Could you check a few things on this model? Use its own coordinates, in mm. Face numbers are marked on the shaded views. A direction names the side the tool comes from. Coordinates: 2 decimals unless noted, no trailing zeros. Write each loop counter-clockwise with the first axis right and the second up, starting at its lowest first coordinate (ties: lowest second). Pieces come first, ordered by that corner, then holes. Notation, with made-up numbers: M -2.5,7 L 38.5,7 A25 ccw 38.5,21 Z; hole C 57,40 d11. An arc over 180 degrees is marked long. Write item = value, one per line.
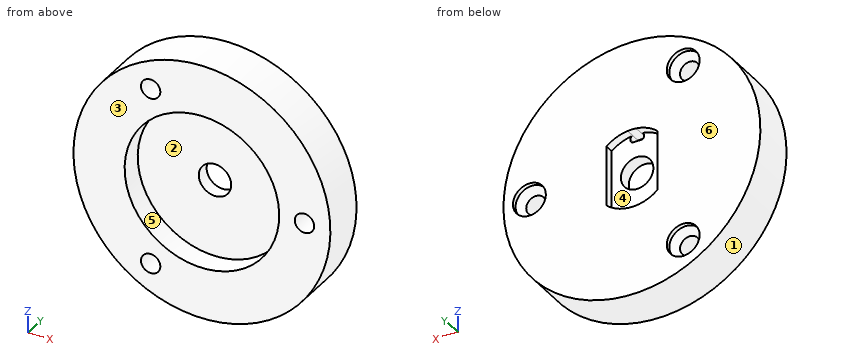
```python
from build123d import *

# Parameters (mm, degrees)
SKETCH_714_R           = 3.6
CUT_EXTRUDE_1503_DEPTH = 2
CUT_EXTRUDE_1558_DEPTH = 4
SKETCH_1765_R          = 2.15
CUT_EXTRUDE_2399_DEPTH = 42.527099586
SKETCH_3_5_R           = 3.65
CUT_EXTRUDE_2433_DEPTH = 0.5
CHAMFER_3010_SIZE      = 2


with BuildPart() as part:
    # Sketch 314 → Повернуть1 (revolve)
    with BuildSketch(Plane.XY, mode=Mode.PRIVATE) as revolve_1_sk:
        Polygon((3.6, 10), (28.5, 10), (28.5, 0), (17.15, 0), (17.15, 5), (3.6, 5), align=None)
    revolve(revolve_1_sk.sketch.rotate(Axis((0, 24.786794377, 0), (0, -1, 0)), 90), axis=Axis((0, 24.786794377, 0), (0, -1, 0)))

    # Sketch 714 → Cut-Extrude 1503 (cut)
    # profile 1 of 2: a face of its own
    with BuildSketch(Plane(origin=(0, 10, 0), x_dir=(1, 0, 0), z_dir=(0, 1, 0))):
        with BuildLine():
            ThreePointArc((-1.5, -7.78), (-1.330121933, -7.369878067), (-0.92, -7.2))
            Line((-0.92, -7.2), (0.92, -7.2))
            ThreePointArc((0.92, -7.2), (1.330121933, -7.369878067), (1.5, -7.78))
            Line((1.5, -7.78), (1.5, -8.082233602))
            ThreePointArc((1.5, -8.082233602), (1.341523495, -8.496233679), (0.947109471, -8.6985909))
            ThreePointArc((0.947109471, -8.6985909), (3.449320455, -8.041435717), (5.65, -6.681317235))
            Line((5.65, -6.681317235), (5.65, 6.681317235))
            ThreePointArc((5.65, 6.681317235), (0, 8.75), (-5.65, 6.681317235))
            Line((-5.65, 6.681317235), (-5.65, -6.681317235))
            ThreePointArc((-5.65, -6.681317235), (-3.449320455, -8.041435717), (-0.947109471, -8.6985909))
            ThreePointArc((-0.947109471, -8.6985909), (-1.341523495, -8.496233679), (-1.5, -8.082233602))
            Line((-1.5, -8.082233602), (-1.5, -7.78))
        make_face()
        with Locations(Location((0, 0, 0), (0, 0, 270))):
            Circle(SKETCH_714_R, mode=Mode.SUBTRACT)
    # profile 2 of 2: a face of its own
    with BuildSketch(Plane(origin=(0, 10, 0), x_dir=(1, 0, 0), z_dir=(0, 1, 0))):
        with BuildLine():
            ThreePointArc((-1.5, -7.78), (-1.330121933, -7.369878067), (-0.92, -7.2))
            Line((-0.92, -7.2), (0.92, -7.2))
            ThreePointArc((0.92, -7.2), (1.330121933, -7.369878067), (1.5, -7.78))
            Line((1.5, -7.78), (1.5, -8.082233602))
            ThreePointArc((1.5, -8.082233602), (1.341523495, -8.496233679), (0.947109471, -8.6985909))
            ThreePointArc((0.947109471, -8.6985909), (0, -8.75), (-0.947109471, -8.6985909))
            ThreePointArc((-0.947109471, -8.6985909), (-1.341523495, -8.496233679), (-1.5, -8.082233602))
            Line((-1.5, -8.082233602), (-1.5, -7.78))
        make_face()
    extrude(amount=-CUT_EXTRUDE_1503_DEPTH, mode=Mode.SUBTRACT)

    # Эскиз2<3> → Cut-Extrude 1558 (cut)
    with BuildSketch(Plane(origin=(0, 10, 0), x_dir=(1, 0, 0), z_dir=(0, 1, 0))):
        with BuildLine():
            ThreePointArc((-1.5, -7.78), (-1.330121933, -7.369878067), (-0.92, -7.2))
            Line((-0.92, -7.2), (0.92, -7.2))
            ThreePointArc((0.92, -7.2), (1.330121933, -7.369878067), (1.5, -7.78))
            Line((1.5, -7.78), (1.5, -8.082233602))
            ThreePointArc((1.5, -8.082233602), (1.341523495, -8.496233679), (0.947109471, -8.6985909))
            ThreePointArc((0.947109471, -8.6985909), (0, -8.75), (-0.947109471, -8.6985909))
            ThreePointArc((-0.947109471, -8.6985909), (-1.341523495, -8.496233679), (-1.5, -8.082233602))
            Line((-1.5, -8.082233602), (-1.5, -7.78))
        make_face()
    extrude(amount=-CUT_EXTRUDE_1558_DEPTH, mode=Mode.SUBTRACT)

    # Sketch 1765 → Cut-Extrude 2399 (cut, through all)
    with BuildSketch(Plane(origin=(0, 10, 0), x_dir=(1, 0, 0), z_dir=(0, 1, 0))):
        with Locations(Location((22.75, 0, 0), (0, 0, 270))):
            Circle(SKETCH_1765_R)
        with Locations(Location((-11.375, -19.702077936, 0), (0, 0, 270))):
            Circle(SKETCH_1765_R)
        with Locations(Location((-11.375, 19.702077936, 0), (0, 0, 270))):
            Circle(SKETCH_1765_R)
    extrude(amount=-CUT_EXTRUDE_2399_DEPTH, mode=Mode.SUBTRACT)

    # Эскиз3<5> → Cut-Extrude 2433 (cut)
    with BuildSketch(Plane(origin=(0, 10, 0), x_dir=(1, 0, 0), z_dir=(0, 1, 0))):
        with Locations(Location((22.75, 0, 0), (0, 0, 270))):
            Circle(SKETCH_3_5_R)
        with Locations(Location((-11.375, -19.702077936, 0), (0, 0, 270))):
            Circle(SKETCH_3_5_R)
        with Locations(Location((-11.375, 19.702077936, 0), (0, 0, 270))):
            Circle(SKETCH_3_5_R)
    extrude(amount=-CUT_EXTRUDE_2433_DEPTH, mode=Mode.SUBTRACT)

    # Chamfer 3010
    # the kernel refuses this chamfer: 2 mm, written as the material it takes off along each edge
    with BuildSketch(Plane(origin=(-11.375, 9.5, -19.702077936), x_dir=(0, 0, 1), z_dir=(-1, 0, 0))) as chamfer_3010_piece_1_section:
        Polygon((2.15 + CHAMFER_3010_SIZE, 0), (2.15, -CHAMFER_3010_SIZE), (2.15, 0), align=None)
    chamfer_3010_piece_1 = revolve(axis=Axis((-11.375, 9.5, -19.702077936), (0, 1, 0)), mode=Mode.PRIVATE)
    chamfer_3010_piece_1 = chamfer_3010_piece_1 & Plane(origin=(-11.375, 8.244810857, -19.702077936), x_dir=(0, 0, 1), z_dir=(0, 1, 0)) * Cylinder(3.65, 17, mode=Mode.PRIVATE)
    add(chamfer_3010_piece_1, mode=Mode.SUBTRACT)
    with BuildSketch(Plane(origin=(22.75, 9.5, 0), x_dir=(0, 0, 1), z_dir=(-1, 0, 0))) as chamfer_3010_piece_2_section:
        Polygon((2.15 + CHAMFER_3010_SIZE, 0), (2.15, -CHAMFER_3010_SIZE), (2.15, 0), align=None)
    chamfer_3010_piece_2 = revolve(axis=Axis((22.75, 9.5, 0), (0, 1, 0)), mode=Mode.PRIVATE)
    chamfer_3010_piece_2 = chamfer_3010_piece_2 & Plane(origin=(22.75, 8.244810857, 0), x_dir=(0, 0, 1), z_dir=(0, 1, 0)) * Cylinder(3.65, 17, mode=Mode.PRIVATE)
    add(chamfer_3010_piece_2, mode=Mode.SUBTRACT)
    with BuildSketch(Plane(origin=(-11.375, 9.5, 19.702077936), x_dir=(0, 0, 1), z_dir=(-1, 0, 0))) as chamfer_3010_piece_3_section:
        Polygon((2.15 + CHAMFER_3010_SIZE, 0), (2.15, -CHAMFER_3010_SIZE), (2.15, 0), align=None)
    chamfer_3010_piece_3 = revolve(axis=Axis((-11.375, 9.5, 19.702077936), (0, 1, 0)), mode=Mode.PRIVATE)
    chamfer_3010_piece_3 = chamfer_3010_piece_3 & Plane(origin=(-11.375, 8.244810857, 19.702077936), x_dir=(0, 0, 1), z_dir=(0, 1, 0)) * Cylinder(3.65, 17, mode=Mode.PRIVATE)
    add(chamfer_3010_piece_3, mode=Mode.SUBTRACT)


solid = part.part
```
Item 1: Imagine slicing it at B-B (z = 0). Write out the boundary of the cut face in (x, y).
Numbers:
outline = M -28.5,0 L -17.15,0 L -17.15,5 L -3.6,5 L -3.6,8 L -5.65,8 L -5.65,10 L -28.5,10 Z; M 3.6,5 L 17.15,5 L 17.15,0 L 20.6,0 L 20.6,7.5 L 19.1,9 L 19.1,10 L 5.65,10 L 5.65,8 L 3.6,8 Z; M 24.9,0 L 28.5,0 L 28.5,10 L 26.4,10 L 26.4,9 L 24.9,7.5 Z
Item 2: Imagine slicing it at C-C (x = -16). Write out the boundary of the cut face in (y, z).
Numbers:
outline = M 0,-23.58 L 10,-23.58 L 10,23.58 L 0,23.58 L 0,6.17 L 5,6.17 L 5,-6.17 L 0,-6.17 Z
Item 3: Imagine slicing it at A-A (x = 0). Write out the boundary of the cut face in (y, z), and give its area (3 significant figures).
Numbers:
outline = M 0,-28.5 L 10,-28.5 L 10,-8.75 L 8,-8.75 L 8,-3.6 L 5,-3.6 L 5,-17.15 L 0,-17.15 Z; M 0,17.15 L 5,17.15 L 5,3.6 L 8,3.6 L 8,7.2 L 6,7.2 L 6,8.75 L 10,8.75 L 10,28.5 L 0,28.5 Z
area = 339 mm²
Item 4: If we mould it in two halves opening along Z, with no side actions, what happens to the marked faces 1, 2, 3 and 4? For each: pulls with the +Z half, pulls with the -Z half, needs draft (parallel to the pull), parting line crosses it, or undercut.
Numbers:
face_1 = parting line crosses it
face_2 = undercut
face_3 = needs draft
face_4 = undercut
Item 5: Imagine slicing it at D-D (y = 2.75). Write out the boundary of the cut face in (x, z) (3 decimals).
Numbers:
outline = C 0,0 d57; hole C 0,0 d34.3; hole C -11.375,-19.702 d4.3; hole C -11.375,19.702 d4.3; hole C 22.75,0 d4.3
Item 6: For the marked faces 5 and 6, which set-ups out of +Z, -Z, +X, -X, +Y, -Y let a thin tool reach every point of the face, with its end or its side?
Numbers:
face_5 = -Y
face_6 = +Z, -Z, +X, -X, +Y
Item 7: I'm going to push flat-ended pins straight in: P1, Ø3.5, axis at x = 22.75, z = 0, coming from the -Y side; P2, Ø5, axis at x = -15.5, y = 3, coming from the -Z side; P3, Ø2, axis at y = 9.5, z = 0.5, coming from the +X side; P4, Ø8.5, axis at x = 0, z = 0, coming from the +Y side. Where does each tip first touch, or does it pass through?
Numbers:
P1 = through
P2 = -25.36
P3 = 28.5
P4 = 8
Item 8: If I drill on line 1 along X through (y, z) = (2.1, 0); line 2 along X through (y, z) = (9.6, 0); line 3 along X through (y, z) = (4, 10), over which ranges is the centre line in solid material (lowest first)?
Numbers:
line_1 = -28.5 to -17.15, 17.15 to 20.6, 24.9 to 28.5
line_2 = -28.5 to -5.65, 5.65 to 19.1, 26.4 to 28.5
line_3 = -26.69 to -13.93, 13.93 to 26.69
